Build history of the part. All positions in model axes, mm. Give positions to 0.01 mm unless a question says otherwise; leave off trailing zeros. Loops run counter-clockwise (first coordinate to the right, second up) from the corner with the lowest first, then second, coordinate; pieces in that order, holes last. Notation, with made-up numbers: (-16, 32.5) - (8, 32.5) arc R25 ccw to (8, 70.5) - close; hole circle Ø9 at (1.25, -13). An arc over 180 degrees is marked (long way). Return JSON: item names as keys, results as strings. Group by question number.
1) Drill centre lines: probe 1 along X at (y, z) = (1.9, -17) (3 decimals); probe 2 along Z at (x, y) = (55.5, 1.3); probe 3 along Z at (x, y) = (-43, 0.7). Where is each one in solid material? Low to high. Write a range as from..to.
2) Drop a flat-ended pin along its axis: pin 1 (1.6 mm diameter, centred on x = -23.5, y = 2, fed in from +Z) (3 decimals). Give the stop position or say it passes through.
3) Slice it at C-C (x = 20). List the corners of the cut face in (y, z) (3 decimals), and give its area (3 significant figures).
4) Slice it at B-B (y = 1.7). Count the separate pieces of the cut face and the enclosed holes in it, and give its area (3 significant figures).
5) Slice it at A-A (z = 23). List the corners of the cut face in (x, y) (3 decimals), and give its area (3 significant figures).
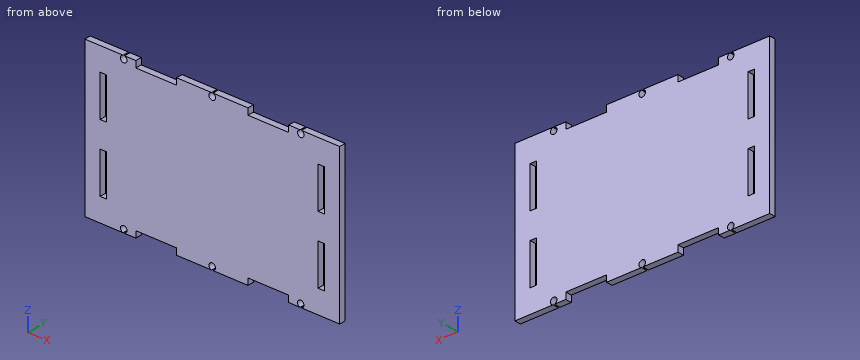
```python
from build123d import *

# Parameters (mm, degrees)
SKETCH1_W           = 127
SKETCH1_H           = 76.2
BOSS_EXTRUDE1_DEPTH = 3.175
SKETCH2_W           = 3.175
SKETCH2_H           = 20.32
CUT_EXTRUDE1_DEPTH  = 3.175
SKETCH3_W           = 20.32
SKETCH3_H           = 3.175
CUT_EXTRUDE2_DEPTH  = 3.175
SKETCH4_R           = 1.6256
CUT_EXTRUDE3_DEPTH  = 3.175


with BuildPart() as part:
    # Sketch1 → Boss-Extrude1 (new body)
    with BuildSketch(Plane(origin=(0, 0, 0), x_dir=(1, 0, 0), z_dir=(0, 1, 0))):
        Rectangle(SKETCH1_W, SKETCH1_H)
    extrude(amount=BOSS_EXTRUDE1_DEPTH)

    # Sketch2 → Cut-Extrude1 (cut)
    with BuildSketch(Plane(origin=(0, 3.175, 0), x_dir=(1, 0, 0), z_dir=(0, 1, 0))):
        with Locations((-54.2925, 16.51)):
            Rectangle(SKETCH2_W, SKETCH2_H)
        with Locations((-54.2925, -16.51)):
            Rectangle(SKETCH2_W, SKETCH2_H)
        with Locations((54.2925, -16.51)):
            Rectangle(SKETCH2_W, SKETCH2_H)
        with Locations((54.2925, 16.51)):
            Rectangle(SKETCH2_W, SKETCH2_H)
    extrude(amount=-CUT_EXTRUDE1_DEPTH, mode=Mode.SUBTRACT)

    # Sketch3 → Cut-Extrude2 (cut)
    with BuildSketch(Plane(origin=(0, 3.175, 0), x_dir=(1, 0, 0), z_dir=(0, 1, 0))):
        with Locations((-27.94, 36.5125)):
            Rectangle(SKETCH3_W, SKETCH3_H)
        with Locations((27.94, 36.5125)):
            Rectangle(SKETCH3_W, SKETCH3_H)
        with Locations((27.94, -36.5125)):
            Rectangle(SKETCH3_W, SKETCH3_H)
        with Locations((-27.94, -36.5125)):
            Rectangle(SKETCH3_W, SKETCH3_H)
    extrude(amount=-CUT_EXTRUDE2_DEPTH, mode=Mode.SUBTRACT)

    # Sketch4 → Cut-Extrude3 (cut)
    with BuildSketch(Plane(origin=(0, 3.175, 0), x_dir=(1, 0, 0), z_dir=(0, 1, 0))):
        with Locations((-44.0944, 36.5125)):
            Circle(SKETCH4_R)
        with Locations((0, 36.5125)):
            Circle(SKETCH4_R)
        with Locations((44.0944, 36.5125)):
            Circle(SKETCH4_R)
        with Locations((44.0944, -36.5125)):
            Circle(SKETCH4_R)
        with Locations((0, -36.5125)):
            Circle(SKETCH4_R)
        with Locations((-44.0944, -36.5125)):
            Circle(SKETCH4_R)
    extrude(amount=-CUT_EXTRUDE3_DEPTH, mode=Mode.SUBTRACT)


solid = part.part
```
Results:
{
 "1": {"probe 1": "-63.5..-55.88, -52.705..52.705, 55.88..63.5", "probe 2": "-38.1..-26.67, -6.35..6.35, 26.67..38.1", "probe 3": "-38.1..-37.71, -35.31..35.31, 37.71..38.1"},
 "2": {"pin 1": "z = 34.925"},
 "3": {"outline": "(0, -34.925) - (3.175, -34.925) - (3.175, 34.925) - (0, 34.925) - close", "area": "222 mm2"},
 "4": {"separate pieces": "1", "enclosed holes": "4", "area": "9,110 mm2"},
 "5": {"outline": "(-63.5, 0) - (-55.88, 0) - (-55.88, 3.175) - (-63.5, 3.175) - close; (-52.705, 0) - (52.705, 0) - (52.705, 3.175) - (-52.705, 3.175) - close; (55.88, 0) - (63.5, 0) - (63.5, 3.175) - (55.88, 3.175) - close", "area": "383 mm2"}
}
